```python
from build123d import *

# Parameters (mm, degrees)
F0_W      = 31.75
F0_H      = 31.75
F0_W_2    = 25.4
F0_H_2    = 25.4
F1_DEPTH  = 1219.2
F2_W      = 25.4
F2_H      = 25.4
F3_DEPTH  = 31.75
F4_R      = 3.81
F5_DEPTH  = 28.576
F7_W      = 25.4
F7_H      = 6.35
F7_H_2    = 31.75
F8_DEPTH  = 25.4
F9_R      = 3.81
F10_DEPTH = 28.576


with BuildPart() as f1:
    # F0 (on Top) → F1 (new body)
    with BuildSketch(Plane.XY):
        Rectangle(F0_W, F0_H)
        Rectangle(F0_W_2, F0_H_2, mode=Mode.SUBTRACT)
    extrude(amount=F1_DEPTH)

    # F7 (on face) → F8 (join)
    with BuildSketch(Plane.YZ.offset(-12.7)):
        with Locations((0, 3.175)):
            Rectangle(F7_W, F7_H)
        with Locations((0, -15.875)):
            Rectangle(F7_W, F7_H_2)
    extrude(amount=F8_DEPTH)

    # F9 (on face) → F10 (cut, through all)
    with BuildSketch(Plane.XZ.offset(12.7)):
        with Locations((0, -12.7)):
            Circle(F9_R)
    extrude(amount=-F10_DEPTH, mode=Mode.SUBTRACT)


with BuildPart() as f3:
    # F2 (on face) → F3 (new body)
    with BuildSketch(Plane(origin=(0, 0, 0), x_dir=(1, 0, 0), z_dir=(0, 0, -1))):
        Rectangle(F2_W, F2_H)
    extrude(amount=F3_DEPTH)

    # F4 (on face) → F5 (cut, through all)
    with BuildSketch(Plane.XZ.offset(12.7)):
        with Locations((0, -12.7)):
            Circle(F4_R)
    extrude(amount=-F5_DEPTH, mode=Mode.SUBTRACT)


solid = f1.part
```
Work out the finished part from the listing and answer in its coordinate system (mm). A direction names the side the tool comes from. Give positions to 0.01 mm unless a question says otherwise; leave off trailing zeros. Order: outer loops, then holes, each group sorted by start corner. A loop starts at its lowest first (then second) coordinate and runs counter-clockwise, first axis right, second up. Notation, with made-up numbers: (-25, 48) - (22, 48) arc R22 ccw to (22, 74) - close; hole circle Ø3 at (43.25, -40). An arc over 180 degrees is marked (long way). One line per item, written item: value. Start each with the question number.
1. Each of these flat-tipped pins is pushed along its axis until it touches: pin 1 Ø1 at (x, y) = (0, -10.5) entering from +Z; pin 2 Ø10 at (x, z) = (0, -12.7) entering from -Y; pin 3 Ø7.5 at (y, z) = (-4.5, -17) entering from +X. Where does it stop, or does it pass through?
2. Section B-B, the plane y = 6 is taken. Write down the section's boundary in (x, z) (3 decimals), then the cut area to 3 significant figures.
3. Which of the six approach directions +Z, -Z, +X, -X, +Y, -Y give full straight-line access (tool end or side, diameter ignored) to faces 5 (the face through (12.7, 0, -16)), 6 (the face through (0, 15.875, 601)), 7 (the face through (-3, 12.7, -16)), 8 (the face through (-14, 0, 1219.2)), 9 (the face through (-12.7, 0, 604))?
4. Section A-A, the plane z = 612.5 is taken. Write down the section's boundary in (x, y) (3 decimals), then the cut area to 3 significant figures.
5. Consider line 1 (Y direction, x = -4, z = 191.5) (3 decimals); line 2 (Z direction, x = 0, y = 0.5). Determine where each line is inside the solid, lowest interval first.
6. For a pull along X with two mould halves and no side action, classify faces 1 (the face through (15.875, 0, 601)), 2 (the face through (0, -12.7, 604)), 3 (the face through (-12.7, 0, -16)), 4 (the face through (3, -12.7, -16)) as released by +X, released by -X, zero draft, split by the parting line, or undercut.
Filled sheet:
1. pin 1: z = 6.35
1. pin 2: y = -12.7
1. pin 3: x = 12.7
2. outline: (-15.875, 0) - (-12.7, 0) - (-12.7, -31.75) - (12.7, -31.75) - (12.7, 0) - (15.875, 0) - (15.875, 1219.2) - (12.7, 1219.2) - (12.7, 6.35) - (-12.7, 6.35) - (-12.7, 1219.2) - (-15.875, 1219.2) - close; hole circle Ø7.62 at (0, -12.7)
2. area: 8,660 mm²
3. face 5: -Z, +X, +Y, -Y
3. face 6: +Z, -Z, +X, -X, +Y
3. face 7: -Z, +X, -X, +Y
3. face 8: +Z, +X, -X, +Y, -Y
3. face 9: +Z
4. outline: (-15.875, -15.875) - (15.875, -15.875) - (15.875, 15.875) - (-15.875, 15.875) - close; hole (-12.7, -12.7) - (12.7, -12.7) - (12.7, 12.7) - (-12.7, 12.7) - close
4. area: 363 mm²
5. line 1: -15.875 to -12.7, 12.7 to 15.875
5. line 2: -31.75 to -16.51, -8.89 to 6.35
6. face 1: released by +X
6. face 2: undercut
6. face 3: released by -X
6. face 4: zero draft
